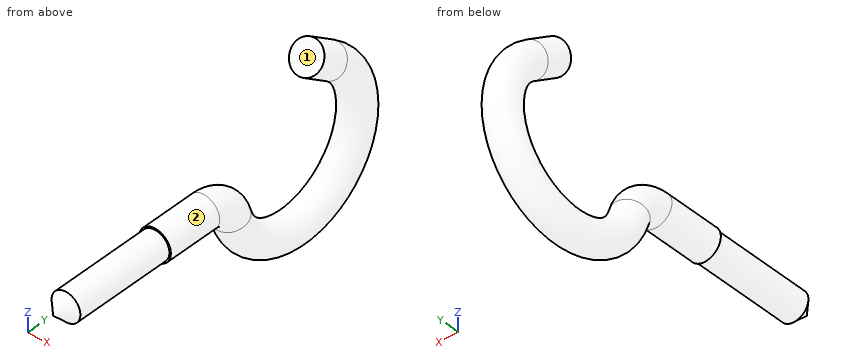
```python
from build123d import *

# Parameters (mm, degrees)
SKETCH001_R  = 2.2
SKETCH002_R  = 2
PAD_DEPTH    = 16
CHAMFER_SIZE = 2


with BuildPart() as part:
    # Sweep: sweep along a path in Sketch
    with BuildLine(Plane.YZ) as sweep_path:
        Line((0, 0), (7.678787, 0))
        ThreePointArc((7.678787, 0), (10.279318, -0.850737), (11.874226, -3.073974))
        ThreePointArc((11.874226, -3.073974), (27.634223, -8.223634), (27.45048, 8.355351))
        Line((27.45048, 8.355351), (23.846219, 10.8791))
    # Sketch001 → Sweep (sweep)
    with BuildSketch(Plane.XZ):
        Circle(SKETCH001_R)
    sweep(path=sweep_path.line, is_frenet=True)

    # Sketch002 → Pad (new body)
    with BuildSketch(Plane.XZ):
        Circle(SKETCH002_R)
    extrude(amount=PAD_DEPTH)

    # Chamfer
    chamfer_edges = [part.edges().sort_by_distance(p)[0] for p in [
        (-2, -16, 0),
    ]]
    chamfer(chamfer_edges, length=CHAMFER_SIZE)


solid = part.part
```
Can you work these out from the model? Positions are in its coordinate system, mm. Face numbers are marked on the shaded views. A direction names the side the tool comes from. Coordinates: 2 decimals unless noted, no trailing zeros. Order: outer loops, then holes, each group sorted by start corner. A loop starts at its lowest first (then second) coordinate and runs counter-clockwise, first axis right, second up. Notation, with made-up numbers: (54.25, 44) -> (67.25, 44) arc R25 ccw to (67.25, 65) -> close; hole circle Ø10 at (44.25, 73.25). An arc over 180 degrees is marked (long way). Write each question's results on one line, items separated by ' | '.
Item 1: I'm going to push flat-ended pins straight in: pin 1 Ø1.5 at (x, z) = (0, 6.5) entering from +Y; pin 2 Ø3 at (y, z) = (25.5, 4) entering from -X. Where does each tip first touch, or does it pass through?
Results are:
pin 1: y = 32.59 | pin 2: through
Item 2: If I drill on line 1 along Y through (x, z) = (1.4, -4); line 2 along Z through (x, y) = (-1.45, 26); line 3 along Y through (x, z) = (0.4, -7), over which ranges is the centre line in solid material (lowest first)?
Results are:
line 1: 10.4 to 14.1, 29.1 to 32.8 | line 2: -11.01 to -7.33, 7.35 to 11.39 | line 3: 11.41 to 17.65, 25.55 to 31.79
Item 3: I want a section at A-A, the plane y = -5. Write out the boundary of the cut face in (x, z).
Results are:
outline: circle Ø4 at (0, 0)
Item 4: Which directions (+Z, -Z, +X, -X, +Y, -Y) give clear straight access to the entire face, cutting with the end or side of a thin tool? Please do the marked faces 1 and 2.
Results are:
face 1: +Z, +X, -X, -Y | face 2: -Y
